Design review of the part built by this model. Coordinates are the model's own, in mm. A direction names the side the tool comes from. Give positions to 0.01 mm unless a question says otherwise; leave off trailing zeros. Order: outer loops, then holes, each group sorted by start corner. A loop starts at its lowest first (then second) coordinate and runs counter-clockwise, first axis right, second up. Notation, with made-up numbers: (80.25, 33) -> (110.25, 33) arc R13 ccw to (110.25, 47) -> close; hole circle Ø11 at (-25, -17.75). An arc over 180 degrees is marked (long way). Use a Markdown table: item, result. Add a question column.
```python
from build123d import *

# Parameters (mm, degrees)
SKETCH1_W           = 875
SKETCH1_H           = 680
BOSS_EXTRUDE1_DEPTH = 210
BOSS_EXTRUDE2_DEPTH = 875
FILLET1_R           = 80


with BuildPart() as part:
    # Sketch1 → Boss-Extrude1 (new body)
    with BuildSketch(Plane(origin=(0, 0, 0), x_dir=(1, 0, 0), z_dir=(0, 1, 0))):
        with Locations((0, 340)):
            Rectangle(SKETCH1_W, SKETCH1_H)
    extrude(amount=-BOSS_EXTRUDE1_DEPTH)

    # Sketch3 → Boss-Extrude2 (add)
    with BuildSketch(Plane.ZY.offset(437.5)):
        Polygon((-70, 0), (-70, 50), (-430, 50), (-480, 0), align=None)
    extrude(amount=-BOSS_EXTRUDE2_DEPTH)

    # Fillet1
    # the kernel refuses this fillet: 80 mm, written as the material it takes off along each edge
    with BuildSketch(Plane(origin=(-622.904962177, 50, -70), x_dir=(0, -1, 0), z_dir=(1, 0, 0))) as fillet1_piece_1:
        with BuildLine():
            CenterArc((80, 74.161984871), FILLET1_R, 180, 67.975687163)
            Line((0, 74.161984871), (-1.6, 74.161984871))
            Line((-1.6, 74.161984871), (-1.6, 0))
            Line((-1.6, 0), (0, -1.6))
            ThreePointArc((0, -1.6), (25, -1.6), (49.4, -1.483239697))
            Line((49.4, -1.483239697), (50, 0))
        make_face()
    extrude(amount=1245.809924355, mode=Mode.SUBTRACT)
    with BuildSketch(Plane(origin=(-520.342712475, 50, -430), x_dir=(0, -0.7071067811865477, -0.7071067811865474), z_dir=(1, 0, 0))) as fillet1_piece_2:
        with BuildLine():
            CenterArc((FILLET1_R * 0.414213562373, -FILLET1_R), FILLET1_R, 90, 45)
            Line((-FILLET1_R * 0.292893218813, -FILLET1_R * 0.292893218813), (-FILLET1_R * 0.307035354437, -FILLET1_R * 0.27875108319))
            Line((-FILLET1_R * 0.307035354437, -FILLET1_R * 0.27875108319), (-FILLET1_R * 0.00828427124746, FILLET1_R * 0.02))
            Line((-FILLET1_R * 0.00828427124746, FILLET1_R * 0.02), (FILLET1_R * 0.414213562373, FILLET1_R * 0.02))
            Line((FILLET1_R * 0.414213562373, FILLET1_R * 0.02), (FILLET1_R * 0.414213562373, 0))
        make_face()
    extrude(amount=1040.685424949, mode=Mode.SUBTRACT)


solid = part.part
```
1) For L1, parallel to Y at x = 366, z = -611.5; L2, parallel to Z at x = -115, y = 5.5; L3, parallel to Z at x = -32.5, y = 3, list the stretches that pass through material, from the lowest coordinate up. Write a range as [from, to].
2) Add section A-A (x = 264.5). Give the boundary of the cut face in (y, z).
3) Machinability: for faces 1 (the flat face through (-6, 0, -581)), 2 (the flat face through (-437.5, -78, -335)), 3 (the flat face through (-6, 0, -35)), which of the approach directions +Z, -Z, +X, -X, +Y, -Y give a long, thin tool a straight path to every point of the face, cutting with its end or side? Answer none if there is none.
4) Insertion check: pin 1 (3 mm diameter, centred on x = -37.5, z = -113, fed in from +Y). The pin has a flat end and moves straight along its axis. Give the tip position at first contact, or say it passes through.
Worked answers:
| question | item | result |
|---|---|---|
| 1 | L1 | [-210, 0] |
| 1 | L2 | [-474.5, -72.47] |
| 1 | L3 | [-477, -71.29] |
| 2 | outline | (-210, -680) -> (0, -680) -> (0, -480) -> (26.57, -453.43) arc R80 ccw to (50, -396.86) -> (50, -144.16) arc R80 ccw to (0, -70) -> (0, 0) -> (-210, 0) -> close |
| 3 | face 1 | -Z, +X, -X, +Y |
| 3 | face 2 | +Z, -Z, -X, +Y, -Y |
| 3 | face 3 | +Z, +X, -X, +Y |
| 4 | pin 1 | y = 44.3 |
